Input: dimensioned drawing with shaded views. Units: mm. Origin: part minimum x, y, z. A direction names the side the tool comes from. Give positions to 0.01 mm unless a question says otherwise; leave off trailing zeros. Write each loop counter-clockwise with the first axis right and the second up, starting at its lowest first coordinate (ties: lowest second). Pieces come first, ordered by that corner, then holes.
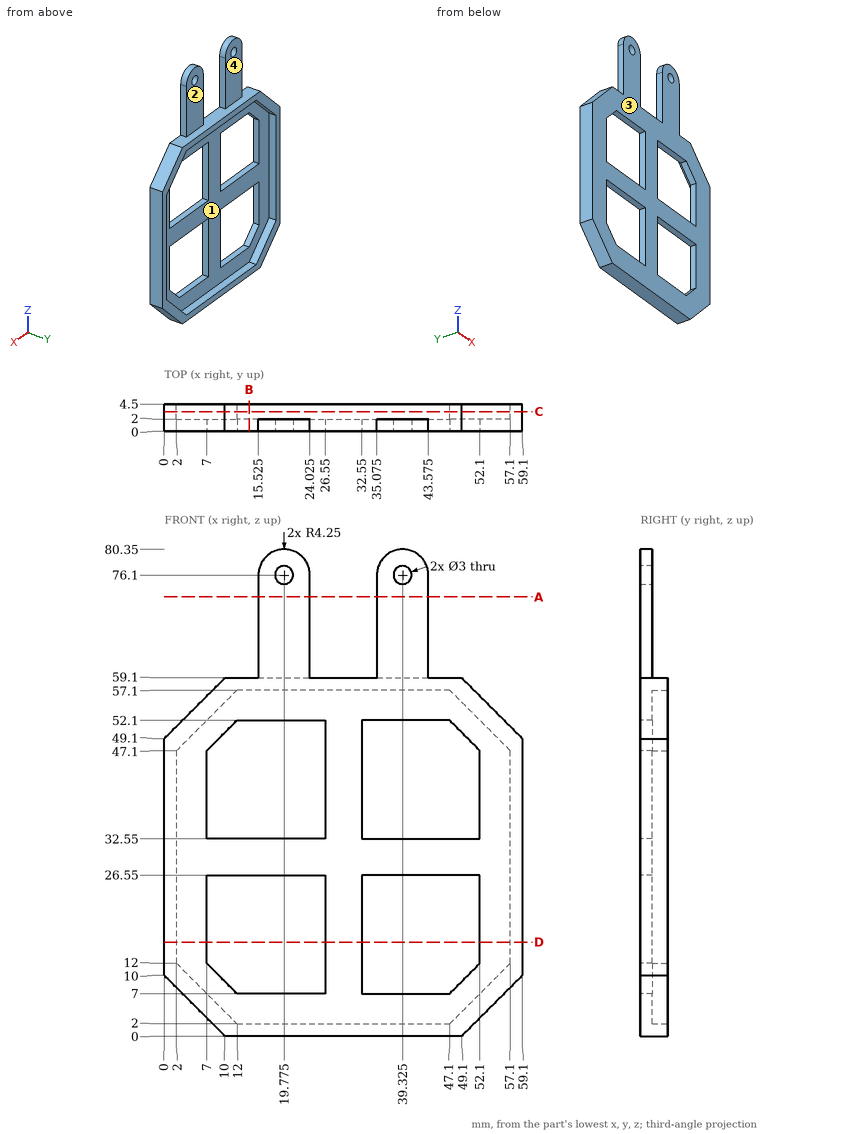
1. Contact query for flat-ended pins moving along their axis: P1, Ø0.6, axis at y = 1, z = 72, coming from the +X side (3 decimals); P2, Ø2, axis at y = 1.5, z = 70.5, coming from the -X side (3 decimals); P3, Ø16.5, axis at x = 43, z = 36, coming from the +Y side; P4, Ø1, axis at y = 4, z = 61, coming from the +X side. Output: stop coordinate, or through.
2. Cut plane B-B, the plane x = 14. Return the cut outline in (y, z), then the cut area to 3 significant figures.
3. Access query for the marked faces 3 and 4. Directions: +Z, -Z, +X, -X, +Y, -Y. A direction counts if a zero-diameter tool reaches every point of the face in a straight line with its end or side. Return the directions, or none.
4. Cut plane A-A, the plane z = 72.5. Return the cut outline in (x, y) (3 decimals).
5. Cut plane C-C, the plane y = 3.25. Return the cut outline in (x, z), then the cut area to 3 significant figures.
6. Line query: L1, parallel to X at y = 1.2, z = 76.1 (3 decimals); L2, parallel to Z at x = 25, y = 1.85; L3, parallel to Z at x = 18, y = 3.85. Output: solid intervals per line, ascending.
7. Mould query, pull axis Z, two halves, no side actions, for the marked faces 1 and 2. Classes: +Z half, -Z half, draft (parallel to the pull), parting line (faces both ways), or undercut.
8. Cut plane D-D, the plane z = 15.5. Return the cut outline in (x, y), then the cut area to 3 significant figures.
Response values:
1. P1: stops at x = 43.575
1. P2: stops at x = 15.525
1. P3: stops at y = 2
1. P4: passes through
2. outline: (0, 0) - (4.5, 0) - (4.5, 2) - (2, 2) - (2, 7) - (0, 7) - close; (0, 26.55) - (2, 26.55) - (2, 32.55) - (0, 32.55) - close; (0, 52.1) - (2, 52.1) - (2, 57.1) - (4.5, 57.1) - (4.5, 59.1) - (0, 59.1) - close
2. area: 50.0 mm2
3. face 3: +Z, -Z, +X, -X, -Y
3. face 4: +Z, +X, -X, +Y
4. outline: (15.525, 0) - (24.025, 0) - (24.025, 2) - (15.525, 2) - close; (35.075, 0) - (43.575, 0) - (43.575, 2) - (35.075, 2) - close
5. outline: (0, 10) - (10, 0) - (49.1, 0) - (59.1, 10) - (59.1, 49.1) - (49.1, 59.1) - (10, 59.1) - (0, 49.1) - close; hole (2, 12) - (12, 2) - (47.1, 2) - (57.1, 12) - (57.1, 47.1) - (47.1, 57.1) - (12, 57.1) - (2, 47.1) - close
5. area: 457 mm2
6. L1: x = 15.525 to 18.275, 21.275 to 24.025, 35.075 to 37.825, 40.825 to 43.575
6. L2: z = 0 to 7, 26.55 to 32.55, 52.1 to 59.1
6. L3: z = 0 to 2, 57.1 to 59.1
7. face 1: undercut
7. face 2: draft
8. outline: (0, 0) - (7, 0) - (7, 2) - (2, 2) - (2, 4.5) - (0, 4.5) - close; (26.55, 0) - (32.55, 0) - (32.55, 2) - (26.55, 2) - close; (52.1, 0) - (59.1, 0) - (59.1, 4.5) - (57.1, 4.5) - (57.1, 2) - (52.1, 2) - close
8. area: 50.0 mm2
